For this review, take the finished solid that the model builds, in its own axes (mm). A direction names the side the tool comes from. Give positions to 0.01 mm unless a question says otherwise; leave off trailing zeros. Order: outer loops, then holes, each group sorted by start corner. A loop starts at its lowest first (then second) coordinate and runs counter-clockwise, first axis right, second up. Notation, with made-up numbers: (27.5, -3) - (55.5, -3) arc R27 ccw to (55.5, 15) - close; hole circle Ø2 at (36, 22.5). An arc over 180 degrees is marked (long way). One line per item, written item: value.
Autodesk Inventor part; units mm, degrees
ref_plane "Work Plane1" through (-2, 13.25, 0) normal (0, 1, 0) x (-1, 0, 0)
ref_plane "YZ Plane" through (0, 0, 0) normal (1, 0, 0) x (0, 1, 0)
ref_plane "XY Plane" through (0, 0, 0) normal (0, 0, 1) x (1, 0, 0)
sketch "Sketch1" plane through (0, 0, 0) normal (0, 1, 0) x (-1, 0, 0)
  line L0 (0, 11.35) -> (0, 12.95)
  line L1 (0.3, 13.25) -> (3.7, 13.25)
  line L2 (0, -11.35) -> (0, -13.25)
  line L3 (0, -13.25) -> (4, -13.25)
  line L4 (4, 12.95) -> (4, 11.25)
  line L5 (4, -13.25) -> (4, -11.25)
  arc A0 (4, 11.25) -> (4, -11.25) centre (34.6406, 0) ccw
  line L6 (0.25, 11.25) -> (0.25, 11.25)
  line L7 (0.25, 11.25) -> (0.25, -11.25)
  line L8 (0.25, -11.25) -> (0.25, -11.25)
  arc A1 (4, 12.95) -> (3.7, 13.25) centre (3.7, 12.95) ccw
  arc A2 (0.3, 13.25) -> (0, 12.95) centre (0.3, 12.95) ccw
  line L9 (0, 11.35) -> (0.25, 11.25)
  line L10 (0, -11.35) -> (0.25, -11.25)
  line L11 (0, 0) -> (3.4534, 0)
  line L12 (2, 0) -> (0.25, 0)
  point P0 (0, 13.25)
  point P1 (4, 13.25)
  point P2 (0, 11.25)
  point P3 (0, -11.25)
  dimension "d0" = 13.25
  dimension "d1" = 26.5
  dimension "d2" = 4
  dimension "d4" = 2
  dimension "d5" = 2
  dimension "d6" = 0.25
  dimension "d7" = 0.3
  dimension "d8" = 0.1
  dimension "d9" = 0.25
  dimension "d10" = 0.1
  dimension "d11" = 0.25
revolve "Revolution1" add sketch "Sketch1" angle 360 about axis through (0, 0, 0) along (-1, 0, 0) contours L0 A2 L1 A1 L4 A0 L11 L7 L9
ref_plane "Work Plane1" through (-2, 13.25, 0) normal (0, 1, 0) x (-1, 0, 0)
sketch "Sketch2" plane through (-2, 13.25, 0) normal (0, 1, 0) x (-1, 0, 0)
  arc A0 (2, 11.25) -> (2, -11.25) centre (32.6406, 0) ccw
  circle A1 centre (0, 0) radius 1
  point P0 (-2, 0)
  dimension "d13" = 2
extrude "Extrusion1" add sketch "Sketch2" along normal blind 2 and the other way blind 1
pattern_circular "Circular Pattern1" count 2 over 360 about axis through (-2, 0, 0) along (-1, 0, 0) of "Extrusion1"
ref_plane "Work Plane2" through (-2, -13.25, 0) normal (0, -1, 0) x (-1, 0, 0)
properties part number "Espejo"
(1) Wall thickness on line 1 (X direction, y = 12.5, z = -4); line 2 (Y direction, x = -1.45, z = 2); line 3 (Y direction, x = -1.3, z = -11): over which ranges is each line inside the solid? List them lowest first. Write a range as from..to.
Answers below:
line 1: x = -3.94..-0.06
line 2: y = -13.1..13.1
line 3: y = -7.39..7.39
(2) Take a section at A-A (z = 0). Write out the cut boundary in (x, y), then the cut area to 3 significant figures.
Answers below:
outline: (-4, -12.95) arc R0.3 ccw to (-3.7, -13.25) - (-3, -13.25) - (-3, -15.25) - (-1, -15.25) - (-1, -13.25) - (-0.3, -13.25) arc R0.3 ccw to (0, -12.95) - (0, -11.35) - (-0.25, -11.25) - (-0.25, 11.25) - (0, 11.35) - (0, 12.95) arc R0.3 ccw to (-0.3, 13.25) - (-1, 13.25) - (-1, 15.25) - (-3, 15.25) - (-3, 13.25) - (-3.7, 13.25) arc R0.3 ccw to (-4, 12.95) - (-4, 11.25) arc R32.64 cw to (-4, -11.25) - close
area: 78.1 mm^2
(3) For P1, Ø1.5, axis at y = -4.5, z = 3.5, coming from the -X side; P2, Ø2, axis at x = -3, y = 0.5, coming from the -Z side; P3, Ø3, axis at y = -5, z = 4.5, coming from the +X side; P4, Ø1.5, axis at x = -0.5, z = -1, coming from the -Y side, all flat-tipped, find the tip position at first contact; note any pin that passes through.
Answers below:
P1: stops at x = -2.64
P2: stops at z = -13.25
P3: stops at x = -0.25
P4: stops at y = -13.25
(4) Draft analysis for pull direction Y (two halves, no side actions). For faces 1 (the face through (-2, -15.25, 0)), 2 (the face through (-2, 15.25, 0)), 3 (the face through (-0.25, 0, 0)), 4 (the face through (-4, 11, -4)), state which applies: pulls with the +Y half, pulls with the -Y half, needs draft (parallel to the pull), parting line crosses it, or undercut.
Answers below:
face 1: pulls with the -Y half
face 2: pulls with the +Y half
face 3: undercut
face 4: needs draft
(5) Machinability: for faces 5 (the face through (0, -11.5, -0.1)), 6 (the face through (-1.2, 14.2, -0.6)), 7 (the face through (-1.2, -14.2, 0.6)), which of the approach directions +Z, -Z, +X, -X, +Y, -Y give a long, thin tool a straight path to every point of the face, cutting with its end or side? Answer none if there is none.
Answers below:
face 5: +Z, -Z, +X, +Y, -Y
face 6: +Y
face 7: -Y
(6) Take a section at B-B (y = 0). Write out the cut boundary in (x, z), then the cut area to 3 significant figures.
Answers below:
outline: (-4, -12.95) arc R0.3 ccw to (-3.7, -13.25) - (-0.3, -13.25) arc R0.3 ccw to (0, -12.95) - (0, -11.35) - (-0.25, -11.25) - (-0.25, 11.25) - (0, 11.35) - (0, 12.95) arc R0.3 ccw to (-0.3, 13.25) - (-3.7, 13.25) arc R0.3 ccw to (-4, 12.95) - (-4, 11.25) arc R32.64 cw to (-4, -11.25) - close
area: 70.1 mm^2
